from build123d import *

# Parameters (mm, degrees)
BASEARM_W             = 8
BASEARM_H             = 40
BOSS_EXTRUDE1_DEPTH   = 3
SKETCH2_R             = 5
SKETCH2_R_2           = 4
BOSS_EXTRUDE2_DEPTH   = 3
BOSS_EXTRUDE3_REACH   = 42.423
SKETCH3_W             = 1
SKETCH3_H             = 3
F_2_0MM_DOWEL_HOLE3_D = 2
SKETCH13_W            = 15
SKETCH13_H            = 7
SKETCH13_R            = 0.5
BOSS_EXTRUDE7_DEPTH   = 3
SKETCH15_W            = 3.5
SKETCH15_H            = 6.077722283
BOSS_EXTRUDE8_DEPTH   = 3
BOSS_EXTRUDE9_START   = -1.95
SKETCH20_R            = 4
SKETCH20_R_2          = 3.5
BOSS_EXTRUDE9_DEPTH   = 1.95
SKETCH16_W            = 4.035898385
SKETCH16_H            = 1
CUT_EXTRUDE5_DEPTH    = 3
BOSS_EXTRUDE10_START  = -4
SKETCH21_R            = 0.5
BOSS_EXTRUDE10_DEPTH  = 4
BOSS_EXTRUDE11_START  = 2
SKETCH22_R            = 0.5
BOSS_EXTRUDE11_DEPTH  = 2
BOSS_EXTRUDE12_DEPTH  = 2
M2_TAPPED_HOLE1_D     = 1.6
M2_TAPPED_HOLE1_DEPTH = 10
M2_TAPPED_HOLE1_TIP   = 0.480688495
CUT_EXTRUDE6_REACH    = 48.992
SKETCH28_R            = 1
BOSS_EXTRUDE13_START  = 3
SKETCH29_R            = 1
BOSS_EXTRUDE13_DEPTH  = 3
BOSS_EXTRUDE14_START  = 0.01
SKETCH30_R            = 1
BOSS_EXTRUDE14_DEPTH  = 0.01
FILLET3_R             = 3
BOSS_EXTRUDE15_START  = -6
BOSS_EXTRUDE15_DEPTH  = 6


with BuildPart() as part:
    # BaseArm → Boss-Extrude1 (new body)
    with BuildSketch(Plane(origin=(0, 0, 0), x_dir=(1, 0, 0), z_dir=(0, 1, 0))):
        with Locations((0, 20)):
            Rectangle(BASEARM_W, BASEARM_H)
    extrude(amount=BOSS_EXTRUDE1_DEPTH)

    # Sketch2 → Boss-Extrude2 (add)
    with BuildSketch(Plane(origin=(0, 0, 0), x_dir=(1, 0, 0), z_dir=(0, 1, 0))):
        with Locations((0, 44)):
            Circle(SKETCH2_R)
        with Locations(Location((0, 44, 0), (0, 0, 270))):
            Circle(SKETCH2_R_2, mode=Mode.SUBTRACT)
    extrude(amount=BOSS_EXTRUDE2_DEPTH)

    # Sketch3 → Boss-Extrude3 (add, up to next)
    with BuildSketch(Plane(origin=(0, 0, -40), x_dir=(-1, 0, 0), z_dir=(0, 0, -1)), mode=Mode.PRIVATE) as boss_extrude3_sk1:
        with Locations((-3.5, 1.5)):
            Rectangle(SKETCH3_W, SKETCH3_H)
    boss_extrude3_tool1 = extrude(boss_extrude3_sk1.sketch, amount=BOSS_EXTRUDE3_REACH, mode=Mode.PRIVATE) - part.part
    # Sketch3 → Boss-Extrude3 (add, up to next)
    with BuildSketch(Plane(origin=(0, 0, -40), x_dir=(-1, 0, 0), z_dir=(0, 0, -1)), mode=Mode.PRIVATE) as boss_extrude3_sk2:
        with Locations((3.5, 1.5)):
            Rectangle(SKETCH3_W, SKETCH3_H)
    boss_extrude3_tool2 = extrude(boss_extrude3_sk2.sketch, amount=BOSS_EXTRUDE3_REACH, mode=Mode.PRIVATE) - part.part
    add(boss_extrude3_tool1.solids().sort_by_distance((3.5, 1.5, -40))[0])
    add(boss_extrude3_tool2.solids().sort_by_distance((-3.5, 1.5, -40))[0])

    # Ø2.0mm Dowel Hole3 (through all)
    with Locations(Plane(origin=(0, 3, -6), x_dir=(0, 0, 1), z_dir=(0, 1, 0))):
        with Locations((0, 0)):
            Hole(F_2_0MM_DOWEL_HOLE3_D / 2)

    # Sketch13 → Boss-Extrude7 (add)
    with BuildSketch(Plane(origin=(0, 3, 0), x_dir=(1, 0, 0), z_dir=(0, 1, 0))):
        with Locations((0, 36.422277717)):
            Rectangle(SKETCH13_W, SKETCH13_H)
        with Locations((-4.375, 36.422277717)):
            Circle(SKETCH13_R, mode=Mode.SUBTRACT)
        with Locations((4.375, 36.422277717)):
            Circle(SKETCH13_R, mode=Mode.SUBTRACT)
    extrude(amount=-BOSS_EXTRUDE7_DEPTH)

    # Sketch15 → Boss-Extrude8 (add)
    with BuildSketch(Plane(origin=(0, 3, 0), x_dir=(1, 0, 0), z_dir=(0, 1, 0))):
        with Locations((-5.75, 42.961138859)):
            Rectangle(SKETCH15_W, SKETCH15_H)
    extrude(amount=-BOSS_EXTRUDE8_DEPTH)

    # Sketch20 → Boss-Extrude9 (add)
    with BuildSketch(Plane(origin=(0, 3, 0), x_dir=(1, 0, 0), z_dir=(0, 1, 0)).offset(BOSS_EXTRUDE9_START)):
        with Locations(Location((0, 44, 0), (0, 0, 270))):
            Circle(SKETCH20_R)
        with Locations(Location((0, 44, 0), (0, 0, 270))):
            Circle(SKETCH20_R_2, mode=Mode.SUBTRACT)
    extrude(amount=BOSS_EXTRUDE9_DEPTH)

    # Sketch16 → Cut-Extrude5 (cut)
    with BuildSketch(Plane(origin=(0, 3, 0), x_dir=(1, 0, 0), z_dir=(0, 1, 0))):
        with Locations((-5.482050808, 44)):
            Rectangle(SKETCH16_W, SKETCH16_H)
    extrude(amount=-CUT_EXTRUDE5_DEPTH, mode=Mode.SUBTRACT)

    # Sketch21 → Boss-Extrude10 (add)
    with BuildSketch(Plane.XZ.offset(BOSS_EXTRUDE10_START)):
        with Locations(Location((-4.375, -36.422277717, 0), (0, 0, 270))):
            Circle(SKETCH21_R)
        with Locations(Location((4.375, -36.422277717, 0), (0, 0, 270))):
            Circle(SKETCH21_R)
    extrude(amount=BOSS_EXTRUDE10_DEPTH)

    # Sketch22 → Boss-Extrude11 (add)
    with BuildSketch(Plane(origin=(0, 4, 0), x_dir=(1, 0, 0), z_dir=(0, 1, 0)).offset(BOSS_EXTRUDE11_START)):
        with Locations(Location((-4.375, 36.422277717, 0), (0, 0, 270))):
            Circle(SKETCH22_R)
    extrude(amount=-BOSS_EXTRUDE11_DEPTH)

    # Sketch23 → Boss-Extrude12 (add)
    with BuildSketch(Plane(origin=(0, 3, 0), x_dir=(1, 0, 0), z_dir=(0, 1, 0))):
        with BuildLine():
            ThreePointArc((-3.172535714, 38.755666806), (-7, 36.422277717), (-3.172535714, 34.088888628))
            ThreePointArc((-3.172535714, 34.088888628), (-3.525, 36.422277717), (-3.172535714, 38.755666806))
        make_face()
    extrude(amount=BOSS_EXTRUDE12_DEPTH)

    # M2 Tapped Hole1
    with Locations(Plane(origin=(0, 0, -46), x_dir=(-1, 0, 0), z_dir=(0, 0, -1))):
        with Locations((6, 1.5)):
            Hole(M2_TAPPED_HOLE1_D / 2, depth=M2_TAPPED_HOLE1_DEPTH)
            with Locations((0, 0, -(M2_TAPPED_HOLE1_DEPTH + M2_TAPPED_HOLE1_TIP / 2))):  # 118° drill point
                Cone(0, M2_TAPPED_HOLE1_D / 2, M2_TAPPED_HOLE1_TIP, mode=Mode.SUBTRACT)

    # Sketch28 → Cut-Extrude6 (cut, up to next)
    with BuildSketch(Plane(origin=(0, 0, -46), x_dir=(-1, 0, 0), z_dir=(0, 0, -1)), mode=Mode.PRIVATE) as cut_extrude6_sk1:
        with Locations((6, 1.5)):
            Circle(SKETCH28_R)
    cut_extrude6_tool1 = extrude(cut_extrude6_sk1.sketch, amount=-CUT_EXTRUDE6_REACH, mode=Mode.PRIVATE) & part.part
    add(cut_extrude6_tool1.solids().sort_by_distance((-6, 1.5, -46))[0], mode=Mode.SUBTRACT)

    # Sketch29 → Boss-Extrude13 (add)
    with BuildSketch(Plane.XZ.offset(BOSS_EXTRUDE13_START)):
        with BuildLine():
            Line((4, -41), (4, -39.922277717))
            Line((4, -39.922277717), (7.5, -39.922277717))
            Line((7.5, -39.922277717), (7.5, -32.922277717))
            Line((7.5, -32.922277717), (4, -32.922277717))
            Line((4, -32.922277717), (4, 0))
            Line((4, 0), (-4, 0))
            Line((-4, 0), (-4, -32.922277717))
            Line((-4, -32.922277717), (-7.5, -32.922277717))
            Line((-7.5, -32.922277717), (-7.5, -43.5))
            Line((-7.5, -43.5), (-3.968626967, -43.5))
            ThreePointArc((-3.968626967, -43.5), (4, -44), (-3.968626967, -44.5))
            Line((-3.968626967, -44.5), (-7.5, -44.5))
            Line((-7.5, -44.5), (-7.5, -46))
            Line((-7.5, -46), (-4.582575695, -46))
            ThreePointArc((-4.582575695, -46), (2.516912515, -48.320318436), (4, -41))
        make_face()
        with Locations(Location((0, -6, 0), (0, 0, 90))):
            Circle(SKETCH29_R, mode=Mode.SUBTRACT)
    extrude(amount=-BOSS_EXTRUDE13_DEPTH)

    # Sketch30 → Boss-Extrude14 (add)
    with BuildSketch(Plane.XZ.offset(3).offset(BOSS_EXTRUDE14_START)):
        with BuildLine():
            Line((4, -16.781929326), (4, 0))
            Line((4, 0), (-4, 0))
            Line((-4, 0), (-4, -16.781929326))
            ThreePointArc((-4, -16.781929326), (0, -17.5), (4, -16.781929326))
        make_face()
        with Locations(Location((0, -6, 0), (0, 0, 90))):
            Circle(SKETCH30_R, mode=Mode.SUBTRACT)
    extrude(amount=-BOSS_EXTRUDE14_DEPTH)

    # Fillet3
    fillet3_edges = [part.edges().sort_by_distance(p)[0] for p in [
        (-4, 0, -32.922277717),
        (4, 0, -32.922277717),
        (4, -0.005, 0),
        (-4, -0.005, 0),
    ]]
    fillet(fillet3_edges, radius=FILLET3_R)

    # Sketch31 → Boss-Extrude15 (add)
    with BuildSketch(Plane(origin=(0, 3, 0), x_dir=(1, 0, 0), z_dir=(0, 1, 0)).offset(BOSS_EXTRUDE15_START)):
        with BuildLine():
            Line((7.332175148, 39.922277717), (4, 39.922277717))
            Line((4, 39.922277717), (4, 41))
            ThreePointArc((4, 41), (4.549561654, 41.925996926), (4.888116765, 42.948185145))
            ThreePointArc((4.888116765, 42.948185145), (5.387339863, 40.851413077), (7.332175148, 39.922277717))
        make_face()
    extrude(amount=BOSS_EXTRUDE15_DEPTH)


solid = part.part
The listing builds one solid part. Answer for the finished solid, in the listing's coordinates (mm). A direction names the side the tool comes from. Coordinates: 2 decimals unless noted, no trailing zeros. Order: outer loops, then holes, each group sorted by start corner. A loop starts at its lowest first (then second) coordinate and runs counter-clockwise, first axis right, second up. Notation, with made-up numbers: M -8.5,2 L 3.5,2 A15 cw 3.5,6 Z; hole C -27,79 d5. An arc over 180 degrees is marked long. Use CSV: the item, a comma, the result in double quotes.
Q1. Straight lines are drawn through the part: L1, parallel to Y at x = 6.5, z = -38; L2, parallel to X at y = -0.65, z = -6; L3, parallel to X at y = 2, z = -41. For each, find the intervals that lie inside material, in ascending order.
Here are the results:
L1,"-3 to 3"
L2,"-4 to -1, 1 to 4"
L3,"-7.5 to -6.62, -5.38 to -1.8, 1.8 to 5.28"
Q2. A tool of negligible diameter and unlimited length cuts with its end or side. For faces 5 (the flat face through (-5, 0, -44.5)), 6 (the cylindrical face through (-5.2, 0.9, -45.3)), 7 (the flat face through (4, 0, -17)), 8 (the flat face through (-4, 0, -16)), 9 (the flat face through (4.4, 4, -36.4)), from which of +Z, -Z, +X, -X, +Y, -Y can it reach the whole face along a straight path? Write none if from no direction.
Here are the results:
face 5,"-X, +Y, -Y"
face 6,"-Z"
face 7,"+Z, +X, +Y, -Y"
face 8,"+Z, -X, +Y, -Y"
face 9,"+Z, -Z, +X, +Y"
Q3. Section A-A (x = 0) is taken. Give the number of separate pieces and of enclosed holes in the cut face, then the cut area to 3 significant figures.
Here are the results:
separate pieces,"3"
enclosed holes,"0"
area,"236 mm2"
Q4. Determine the mould class of faces 1 (the flat face through (-7.5, 0, -38)), 2 (the cylindrical face through (-4.855, -0.042, -32.02)), 3 (the flat face through (-6, 0, -43.5)), 4 (the cylindrical face through (5.368, -0.042, -40.876)) for opening direction Z: pulls with the +Z half, pulls with the -Z half, needs draft (parallel to the pull), parting line crosses it, or undercut.
Here are the results:
face 1,"needs draft"
face 2,"pulls with the +Z half"
face 3,"undercut"
face 4,"undercut"
Q5. Section C-C (y = -1.5) is taken. Determine the outline of the cut face in (x, z).
Here are the results:
outline,"M -7.5,-46 L -4.58,-46 A5 ccw 4.89,-42.95 A2.5 cw 7.33,-39.92 L 7.5,-39.92 L 7.5,-32.92 L 7,-32.92 A3 cw 4,-29.92 L 4,-3 A3 ccw 1,0 L -1,0 A3 ccw -4,-3 L -4,-29.92 A3 cw -7,-32.92 L -7.5,-32.92 L -7.5,-43.5 L -3.97,-43.5 A4 cw long -3.97,-44.5 L -7.5,-44.5 Z; hole C 0,-6 d2"
Q6. Section B-B (z = -42.5) is taken. Determine the outline of the cut face in (x, y), then the cut area to 3 significant figures.
Here are the results:
outline,"M -7.5,-3 L -3.71,-3 L -3.71,1.05 L -3.16,1.05 L -3.16,3 L -7.5,3 Z; M 3.16,1.05 L 3.71,1.05 L 3.71,-3 L 4.83,-3 L 4.83,3 L 3.16,3 Z; hole C -6,1.5 d1.6"
area,"29.6 mm2"
Q7. Given pin 1 Ø1 at (x, y) = (-6, 1.5) entering from -Z; pin 2 Ø3 at (x, z) = (0, -6) entering from -Y; pin 3 Ø2 at (y, z) = (2, -13) entering from +X; pin 4 Ø0.6 at (x, y) = (-7, 1) entering from +Z, each flat-ended and moving along its own axis, determine where each tip first touches the part or whether it passes through.
Here are the results:
pin 1,"z = -35.82"
pin 2,"y = -3.01"
pin 3,"x = 4"
pin 4,"z = -32.91"
Q8. Section D-D (y = 3.5) is taken. Determine the outline of the cut face in (x, z) (3 decimals), then the cut area to 3 significant figures.
Here are the results:
outline,"M -3.173,-38.756 A7.9 cw -3.173,-34.089 A2.625 ccw long Z; C 4.375,-36.422 d1"
area,"16.6 mm2"
